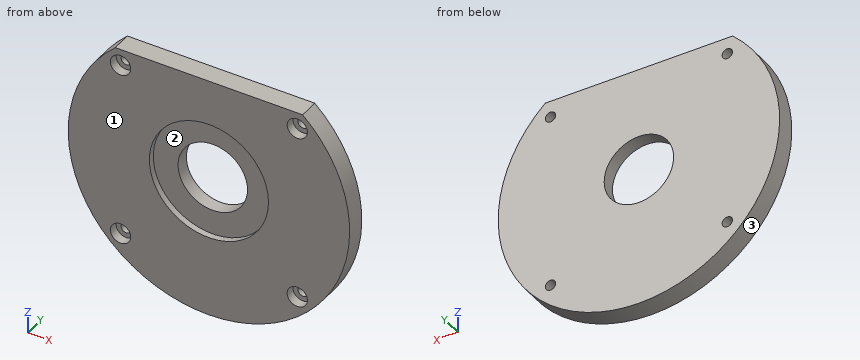
```python
from build123d import *

# Parameters (mm, degrees)
F0_R           = 44.9961
F0_R_2         = 11.1125
F1_DEPTH       = 6.35
F2_R           = 19.05
F3_DEPTH       = 2.032
F5_D           = 3.3
F5_CBORE_D     = 6.5
F5_CBORE_DEPTH = 3
F7_DEPTH       = 25.4


with BuildPart() as f1:
    # F0 (on Front) → F1 (new body)
    with BuildSketch(Plane.XZ):
        Circle(F0_R)
        Circle(F0_R_2, mode=Mode.SUBTRACT)
    extrude(amount=F1_DEPTH)

    # F2 (on face) → F3 (cut)
    with BuildSketch(Plane.XZ.offset(6.35)):
        Circle(F2_R)
    extrude(amount=-F3_DEPTH, mode=Mode.SUBTRACT)

    # F5 (through all)
    with Locations(Plane.XZ.offset(6.35)):
        with Locations((-28.2702, 28.2702), (28.2702, 28.2702), (28.2702, -28.2702), (-28.2702, -28.2702)):
            CounterBoreHole(F5_D / 2, F5_CBORE_D / 2, F5_CBORE_DEPTH)

    # F6 (on face) → F7 (cut)
    with BuildSketch(Plane.XZ.offset(6.35)):
        with BuildLine():
            ThreePointArc((29.9660799238, 33.5661), (0, 44.9961), (-29.9660799238, 33.5661))
            Line((-29.9660799238, 33.5661), (29.9660799238, 33.5661))
        make_face()
    extrude(amount=-F7_DEPTH, mode=Mode.SUBTRACT)


solid = f1.part
```
Verification items for the finished model (mm, model axes). Face numbers are marked on the shaded views. Give positions to 0.01 mm unless a question says otherwise; leave off trailing zeros. Order: outer loops, then holes, each group sorted by start corner. A loop starts at its lowest first (then second) coordinate and runs counter-clockwise, first axis right, second up. Notation, with made-up numbers: M 52,28.5 L 64,28.5 A17 cw 64,59.5 Z; hole C 71.5,12 d2. An arc over 180 degrees is marked long. Answer in a Markdown table with one row per item. Add a question column.
Item 1: Scan lines: probe 1 along Z at (x, y) = (30.5, -5); probe 2 along Z at (x, y) = (26, -5); probe 3 along Z at (x, y) = (0, -4.8). Record each from-to range of solid material in increasing order. Write a range as from..to.
Item 2: Section check A-A, the plane x = 0. Enter the section's corners in (y, z).
Item 3: Section check D-D, the plane z = 15.5. Enter the section's corners in (x, y).
Item 4: Section check C-C, the plane x = -28. Enter the section's corners in (y, z), and give its area (3 significant figures).
Item 5: Section check B-B, the plane z = 0. Enter the section's corners in (x, y), and give its area (3 significant figures).
Item 6: Gauge pin test, flat ends, axial feed: pin 1 (3 mm diameter, centred on y = -4, z = 3, fed in from -X); pin 2 (5.5 mm diameter, centred on x = 28.27, z = -28.27, fed in from -Y); pin 3 (3 mm diameter, centred on y = -2, z = 8.5, fed in from +X). Record the tip position at first contact, or that the pin passes through.
Item 7: Mould release check, pull along X, two halves, no side actions. Record for the marked faces 1, 2 and 3: released by +X, released by -X, zero draft, split by the parting line, or undercut.
Filled sheet:
| question | item | result |
|---|---|---|
| 1 | probe 1 | z = -33.08..-30.63, -25.91..25.91, 30.63..33.08 |
| 1 | probe 2 | z = -36.72..-30.6, -25.94..25.94, 30.6..33.57 |
| 1 | probe 3 | z = -45..-19.05, 19.05..33.57 |
| 2 | outline | M -6.35,-45 L 0,-45 L 0,-11.11 L -4.32,-11.11 L -4.32,-19.05 L -6.35,-19.05 Z; M -6.35,19.05 L -4.32,19.05 L -4.32,11.11 L 0,11.11 L 0,33.57 L -6.35,33.57 Z |
| 3 | outline | M -42.24,-6.35 L -11.07,-6.35 L -11.07,-4.32 L 11.07,-4.32 L 11.07,-6.35 L 42.24,-6.35 L 42.24,0 L -42.24,0 Z |
| 4 | outline | M -6.35,-35.22 L 0,-35.22 L 0,-29.9 L -3.35,-29.9 L -3.35,-31.51 L -6.35,-31.51 Z; M -6.35,-25.03 L -3.35,-25.03 L -3.35,-26.64 L 0,-26.64 L 0,26.64 L -3.35,26.64 L -3.35,25.03 L -6.35,25.03 Z; M -6.35,31.51 L -3.35,31.51 L -3.35,29.9 L 0,29.9 L 0,33.57 L -6.35,33.57 Z |
| 4 | area | 376 mm^2 |
| 5 | outline | M -45,-6.35 L -19.05,-6.35 L -19.05,-4.32 L -11.11,-4.32 L -11.11,0 L -45,0 Z; M 11.11,-4.32 L 19.05,-4.32 L 19.05,-6.35 L 45,-6.35 L 45,0 L 11.11,0 Z |
| 5 | area | 398 mm^2 |
| 6 | pin 1 | stops at x = -44.97 |
| 6 | pin 2 | stops at y = -3.35 |
| 6 | pin 3 | stops at x = 44.45 |
| 7 | face 1 | zero draft |
| 7 | face 2 | undercut |
| 7 | face 3 | split by the parting line |
